Job drawing, mm, ordinate dimensions from the low corner. One solid piece. Round coordinates to 2 decimals unless told otherwise and drop trailing zeros. Order: outer loops, then holes, each group sorted by start corner. A loop starts at its lowest first (then second) coordinate and runs counter-clockwise, first axis right, second up. Notation, with made-up numbers: M 28,50.25 L 48,50.25 A17 cw 48,75.25 Z; hole C 21.5,64 d5. An arc over 180 degrees is marked long. Answer as a JSON object with one key per item and string values. Group by question number.
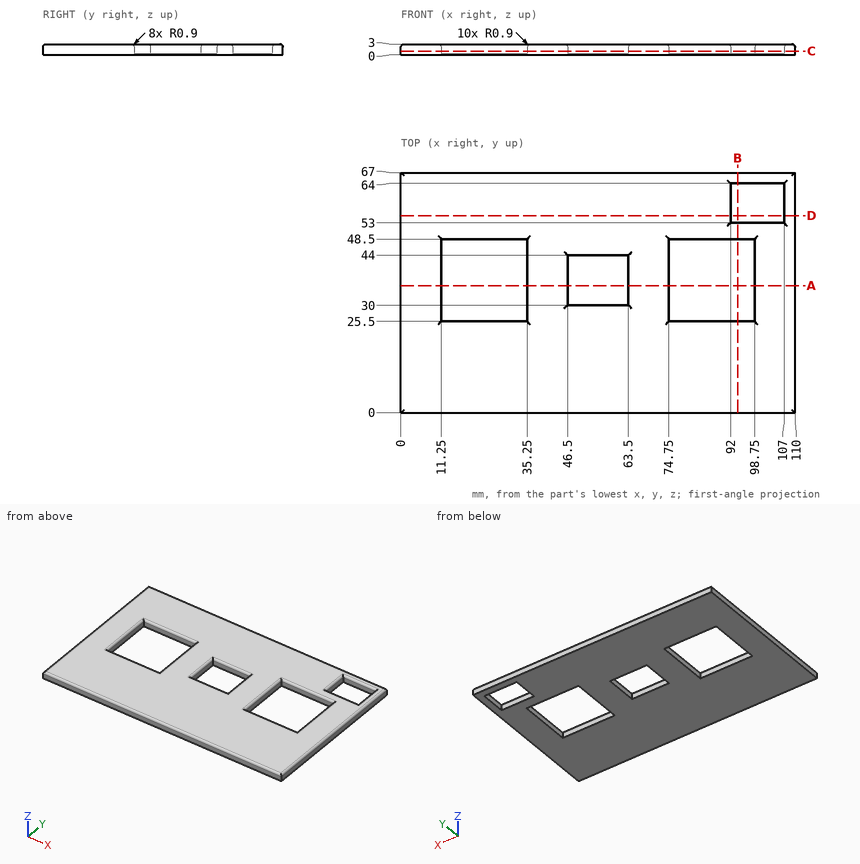
Item 1: Cut at A-A, the plane y = 35.5. Give the cut face in (x, z).
Item 2: Cut at D-D, the plane y = 55. Give the cut face in (x, z).
Item 3: Cut at C-C, the plane z = 1. Give the cut face in (x, y).
Item 4: Cut at B-B, the plane x = 94. Give the cut face in (y, z).
Item 5: Drill centre lines: line 1 (X direction, y = 40, z = 1.4); line 2 (X direction, y = 26, z = 0.2). Where is each one in solid material? Low to high. Write a range as [from, to].
Item 6: Flat gauge pin, fed straight in: pin 1 Ø8 at (x, y) = (78, 45.5) entering from -Z. Where does the tip first touch, or does it go through?
Response values:
{
 "1": {"outline": "M 0,0 L 11.25,0 L 11.25,2.1 A0.9 ccw 10.35,3 L 0.9,3 A0.9 ccw 0,2.1 Z; M 35.25,0 L 46.5,0 L 46.5,2.1 A0.9 ccw 45.6,3 L 36.15,3 A0.9 ccw 35.25,2.1 Z; M 63.5,0 L 74.75,0 L 74.75,2.1 A0.9 ccw 73.85,3 L 64.4,3 A0.9 ccw 63.5,2.1 Z; M 98.75,0 L 110,0 L 110,2.1 A0.9 ccw 109.1,3 L 99.65,3 A0.9 ccw 98.75,2.1 Z"},
 "2": {"outline": "M 0,0 L 92,0 L 92,2.1 A0.9 ccw 91.1,3 L 0.9,3 A0.9 ccw 0,2.1 Z; M 107,0 L 110,0 L 110,2.1 A0.9 ccw 109.1,3 L 107.9,3 A0.9 ccw 107,2.1 Z"},
 "3": {"outline": "M 0,0 L 110,0 L 110,67 L 0,67 Z; hole M 11.25,25.5 L 35.25,25.5 L 35.25,48.5 L 11.25,48.5 Z; hole M 46.5,30 L 63.5,30 L 63.5,44 L 46.5,44 Z; hole M 74.75,25.5 L 98.75,25.5 L 98.75,48.5 L 74.75,48.5 Z; hole M 92,53 L 107,53 L 107,64 L 92,64 Z"},
 "4": {"outline": "M 0,0 L 25.5,0 L 25.5,2.1 A0.9 ccw 24.6,3 L 0.9,3 A0.9 ccw 0,2.1 Z; M 48.5,0 L 53,0 L 53,2.1 A0.9 ccw 52.1,3 L 49.4,3 A0.9 ccw 48.5,2.1 Z; M 64,0 L 67,0 L 67,2.1 A0.9 ccw 66.1,3 L 64.9,3 A0.9 ccw 64,2.1 Z"},
 "5": {"line 1": "[0, 11.25], [35.25, 46.5], [63.5, 74.75], [98.75, 110]", "line 2": "[0, 11.25], [35.25, 74.75], [98.75, 110]"},
 "6": {"pin 1": "z = 0"}
}
